Here's how the part is built. I have some questions about the finished solid (model axes, mm). Round coordinates to 2 decimals unless told otherwise and drop trailing zeros. One line per question, with ' | ' between items. Start each with the question number.
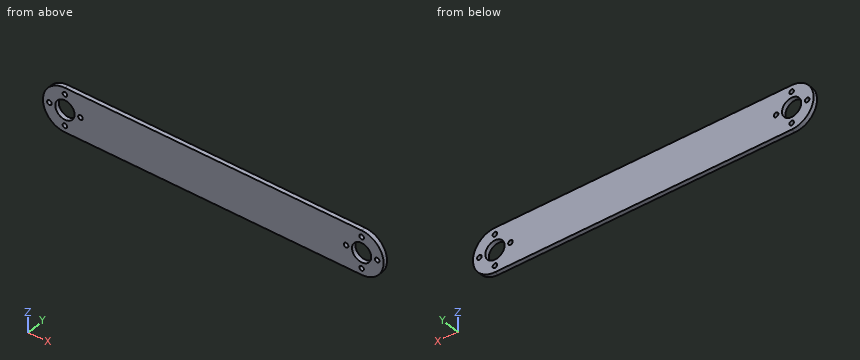
```python
from build123d import *

# Parameters (mm, degrees)
SKETCH1_R           = 7
BOSS_EXTRUDE1_DEPTH = 3.175
SKETCH2_R           = 1.65
CUT_EXTRUDE1_DEPTH  = 10


with BuildPart() as part:
    # Sketch1 → Boss-Extrude1 (new body)
    with BuildSketch(Plane(origin=(0, 0, 0), x_dir=(1, 0, 0), z_dir=(0, 1, 0))):
        with BuildLine():
            Line((0, 0), (216, 0))
            ThreePointArc((216, 0), (232, 16), (216, 32))
            Line((216, 32), (0, 32))
            ThreePointArc((0, 32), (-16, 16), (0, 0))
        make_face()
        with Locations(Location((0, 16, 0), (0, 0, 270))):
            Circle(SKETCH1_R, mode=Mode.SUBTRACT)
        with Locations(Location((216, 16, 0), (0, 0, 270))):
            Circle(SKETCH1_R, mode=Mode.SUBTRACT)
    extrude(amount=BOSS_EXTRUDE1_DEPTH)

    # Sketch2 → Cut-Extrude1 (cut)
    with BuildSketch(Plane(origin=(0, 3.175, 0), x_dir=(1, 0, 0), z_dir=(0, 1, 0))):
        with Locations(Location((204.686291501, 16, 0), (0, 0, 270))):
            Circle(SKETCH2_R)
        with Locations(Location((216, 27.313708499, 0), (0, 0, 270))):
            Circle(SKETCH2_R)
        with Locations(Location((-11.313708499, 16, 0), (0, 0, 270))):
            Circle(SKETCH2_R)
        with Locations(Location((0, 27.313708499, 0), (0, 0, 270))):
            Circle(SKETCH2_R)
        with Locations(Location((11.313708499, 16, 0), (0, 0, 270))):
            Circle(SKETCH2_R)
        with Locations(Location((0, 4.686291501, 0), (0, 0, 270))):
            Circle(SKETCH2_R)
        with Locations(Location((216, 4.686291501, 0), (0, 0, 270))):
            Circle(SKETCH2_R)
        with Locations(Location((227.313708499, 16, 0), (0, 0, 270))):
            Circle(SKETCH2_R)
    extrude(amount=-CUT_EXTRUDE1_DEPTH, mode=Mode.SUBTRACT)


solid = part.part
```
1) I'm going to push flat-ended pins straight in: pin 1 Ø2 at (x, z) = (11.31, -16) entering from +Y; pin 2 Ø1 at (y, z) = (2, -17.5) entering from +X. Where does each tip first touch, or does it pass through?
2) Please list where these lines run through material, in increasing order: L1, parallel to Z at x = 216.5, y = 0.6; L2, parallel to X at y = 1.45, z = -18.5; L3, parallel to X at y = 2.3, z = -22. Write a range as from..to.
3) Imagine slicing it at A-A (y = 1.75). State how many separate pieces and enclosed holes the cut face has, then the cut area to 3 significant figures.
Results are:
1) pin 1: through | pin 2: x = 231.97
2) L1: -31.99..-28.89, -25.74..-22.98, -9.02..-6.26, -3.11..-0.01 | L2: -15.8..-6.54, 6.54..209.46, 222.54..231.8 | L3: -14.83..-3.61, 3.61..212.39, 219.61..230.83
3) separate pieces: 1 | enclosed holes: 10 | area: 7,340 mm²
